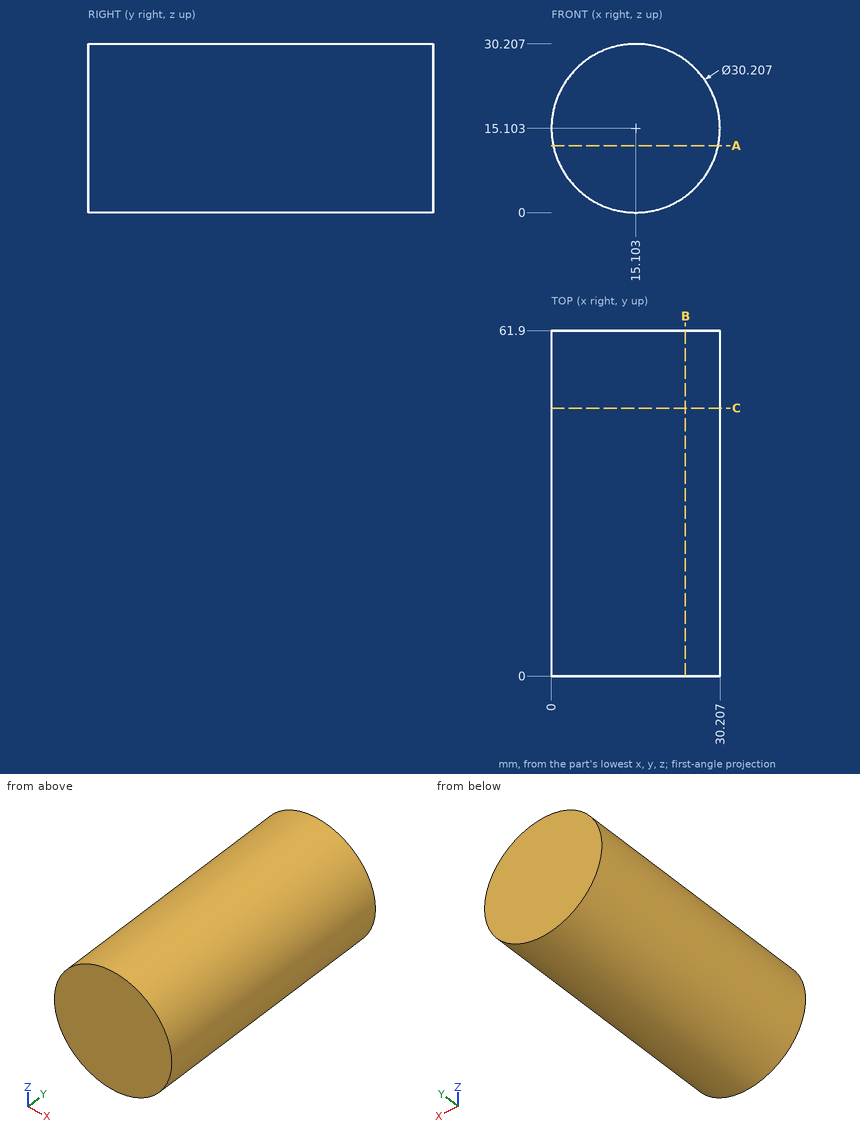
Geometry check sheet. Reference: drawing and pictorial views, mm from the part's lowest x, y, z. Round coordinates to 2 decimals unless told otherwise and drop trailing zeros. Write each loop counter-clockwise with the first axis right and the second up, starting at its lowest first coordinate (ties: lowest second). Pieces come first, ordered by that corner, then holes.
(1) Depth check by flat-ended pin: pin 1 Ø1 at (x, y) = (11, 41.5) entering from -Z; pin 2 Ø2 at (y, z) = (16.5, 8) entering from -X; pin 3 Ø2 at (x, y) = (12.5, 21) entering from +Z. Enter the tip coordinate at first touch or a pass-through.
Returned:
pin 1: stops at z = 0.44
pin 2: stops at x = 1.29
pin 3: stops at z = 30.12
(2) Section check B-B (x = 24). Enter the section's corners in (y, z), plus the area to 3 significant figures.
Returned:
outline: (0, 2.9) - (61.9, 2.9) - (61.9, 27.31) - (0, 27.31) - close
area: 1,510 mm2
(3) Section check C-C (y = 48). Enter the section's corners in (x, z).
Returned:
outline: circle Ø30.21 at (15.1, 15.1)
(4) Section check A-A (z = 12). Enter the section's corners in (x, y) (1 decimal), plus the area to 3 significant figures.
Returned:
outline: (0.3, 0) - (29.9, 0) - (29.9, 61.9) - (0.3, 61.9) - close
area: 1,830 mm2
(5) Material ranges on line 1 (X direction, y = 26, z = 15); line 2 (Z direction, x = 9, y = 14.5); line 3 (X direction, y = 54, z = 23), recorded low to high.
Returned:
line 1: x = 0 to 30.21
line 2: z = 1.29 to 28.92
line 3: x = 2.23 to 27.98
